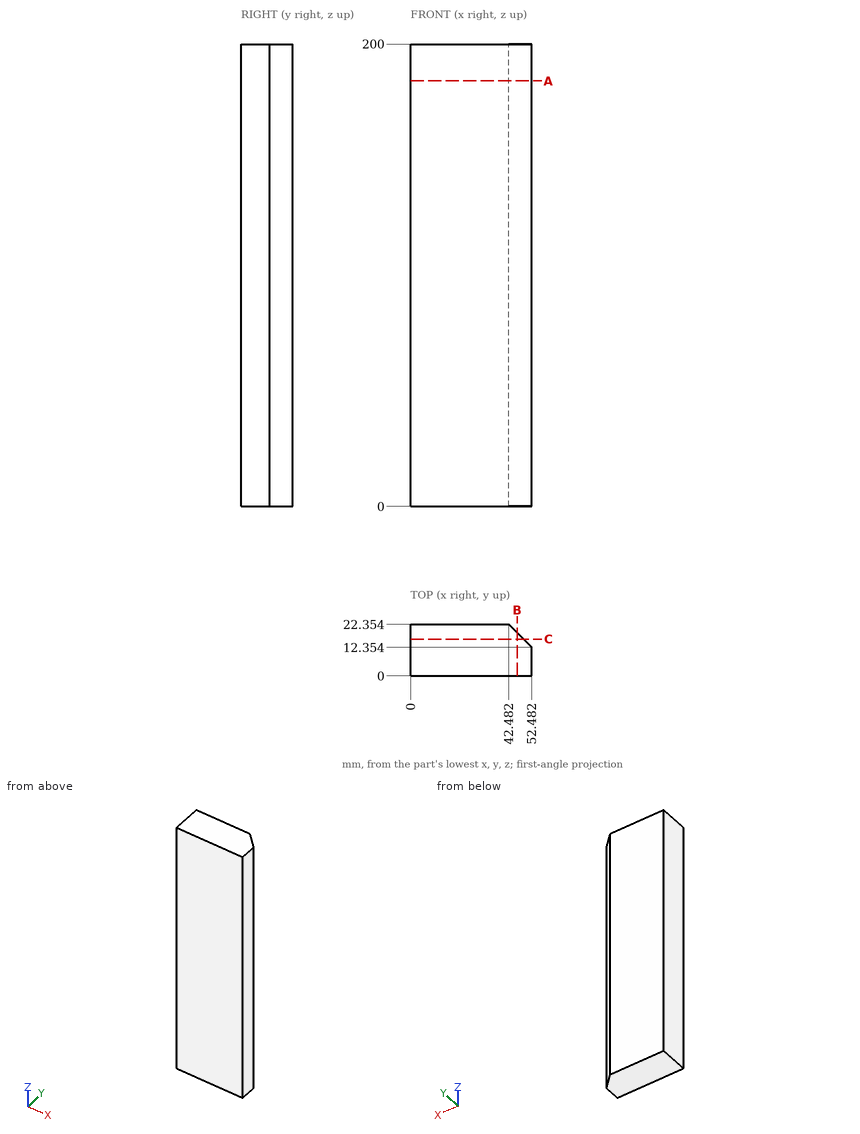
Verification items for this drawing (mm, ordinates from the low corner). Round coordinates to 2 decimals unless told otherwise and drop trailing zeros. Order: outer loops, then holes, each group sorted by start corner. A loop starts at its lowest first (then second) coordinate and runs counter-clockwise, first axis right, second up. Notation, with made-up numbers: (85, 29) - (128, 29) arc R36 ccw to (128, 67) - close; hole circle Ø4 at (79, 3.25). An arc over 180 degrees is marked (long way). Answer as CSV lines item,"result". Start each with the question number.
1) Section check C-C (y = 16). Record the cut outline in (x, z).
2) Section check A-A (z = 184). Record the cut outline in (x, y).
3) Scan lines: probe 1 along X at (y, z) = (17.25, 32) (1 decimal); probe 2 along Y at (x, z) = (46, 150) (1 decimal); probe 3 along X at (y, z) = (19, 121) (1 decimal). Record each from-to range of solid material in increasing order.
4) Section check B-B (x = 46). Record the cut outline in (y, z), then the cut area to 3 significant figures.
Determined:
1,outline,"(0, 0) - (48.84, 0) - (48.84, 200) - (0, 200) - close"
2,outline,"(0, 0) - (52.48, 0) - (52.48, 12.35) - (42.48, 22.35) - (0, 22.35) - close"
3,probe 1,"0 to 47.6"
3,probe 2,"0 to 18.8"
3,probe 3,"0 to 45.8"
4,outline,"(0, 0) - (18.84, 0) - (18.84, 200) - (0, 200) - close"
4,area,"3,770 mm^2"
